Read the model definition and answer for the solid it produces. Units are mm, in the model's axes. Face numbers are marked on the shaded views. Coordinates: 2 decimals unless noted, no trailing zeros. Loops run counter-clockwise (first coordinate to the right, second up) from the corner with the lowest first, then second, coordinate; pieces in that order, holes last. Notation, with made-up numbers: M -37,51.25 L -14,51.25 A28 ccw -14,88.25 Z; hole C 46.5,85.5 d10. An arc over 180 degrees is marked long. One line per item, written item: value. Start each with the question number.
1. Determine the mould class of the marked faces 1, 2 and 3 for opening direction X: +X half, -X half, draft (parallel to the pull), parting line (faces both ways), or undercut.
2. The part is cut by section C-C (x = 20). Write down the section's boundary in (y, z).
3. The part is cut by section B-B (x = 65). Write down the section's boundary in (y, z), then the cut area to 3 significant figures.
4. The part is cut by section A-A (y = 1). Write down the section's boundary in (x, z), then the cut area to 3 significant figures.
5. Flat-ended cylindrical pins translate along their axes: pin 1 (1.5 mm diameter, centred on x = 39.5, y = 3.5, fed in from +Z); pin 2 (0.5 mm diameter, centred on y = 1, z = -0.5, fed in from +X); pin 3 (4.5 mm diameter, centred on x = 84.5, z = 7.5, fed in from -Y); pin 4 (5.5 mm diameter, centred on x = 0, z = 0, fed in from +Y). Find the tip coordinate at first contact, or state that the pin passes through.
6. Consider probe 1 along X at (y, z) = (0.75, 4); probe 2 along X at (y, z) = (0.5, 5.5); probe 3 along Y at (x, z) = (1, -3). Determine where each line is inside the solid, lowest interval first.
7. The part is cut by section D-D (z = 9.5). Write down the section's boundary in (x, y), then the cut area to 3 significant figures.
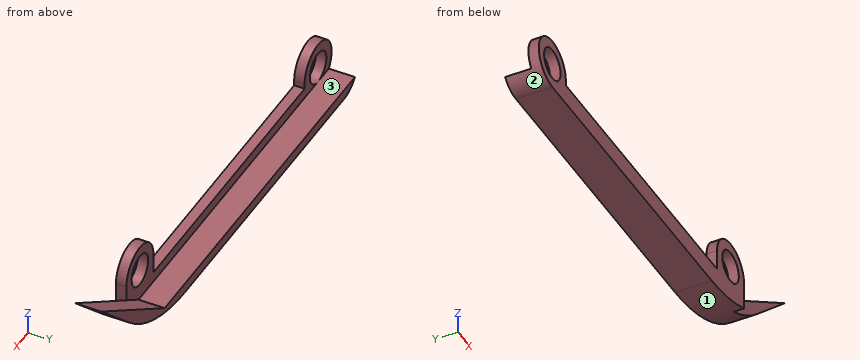
```python
from build123d import *

# Parameters (mm, degrees)
SKETCH1_R           = 3.06
BOSS_EXTRUDE1_DEPTH = 2
BOSS_EXTRUDE2_START = -2
BOSS_EXTRUDE2_DEPTH = 5
SKETCH6_W           = 56
SKETCH6_H           = 2
BOSS_EXTRUDE3_DEPTH = 2
FILLET1_R           = 30
FILLET2_R           = 5


with BuildPart() as part:
    # Sketch1 → Boss-Extrude1 (new body)
    with BuildSketch(Plane(origin=(0, 0, 0), x_dir=(1, 0, 0), z_dir=(0, 1, 0))):
        with BuildLine():
            Line((-5, 0), (-5, 5))
            Line((-5, 5), (71, 5))
            Line((71, 5), (71, -3))
            ThreePointArc((71, -3), (66, -8), (61, -3))
            Line((61, -3), (61, 3.06))
            Line((61, 3.06), (5, 3.06))
            Line((5, 3.06), (5, 0))
            ThreePointArc((5, 0), (0, -5), (-5, 0))
        make_face()
        with Locations(Location((0, 0, 0), (0, 0, 270))):
            Circle(SKETCH1_R, mode=Mode.SUBTRACT)
        with Locations(Location((66, -3, 0), (0, 0, 270))):
            Circle(SKETCH1_R, mode=Mode.SUBTRACT)
    extrude(amount=BOSS_EXTRUDE1_DEPTH)

    # Sketch4 → Boss-Extrude2 (add)
    with BuildSketch(Plane(origin=(0, 0, 0), x_dir=(-1, 0, 0), z_dir=(0, -1, 0)).offset(BOSS_EXTRUDE2_START)):
        Polygon((5, 5), (-71, 5), (-90, -13.010835443), (-66.5, 3.06), (5, 3.06), align=None)
    extrude(amount=-BOSS_EXTRUDE2_DEPTH)

    # Sketch6 → Boss-Extrude3 (add)
    with BuildSketch(Plane(origin=(0, 0, 0), x_dir=(-1, 0, 0), z_dir=(0, -1, 0))):
        with Locations((-33, 2.06)):
            Rectangle(SKETCH6_W, SKETCH6_H)
    extrude(amount=-BOSS_EXTRUDE3_DEPTH)

    # Fillet1
    # the kernel refuses this fillet: 30 mm, written as the material it takes off along each edge
    with BuildSketch(Plane(origin=(71, -27.8984931, -5), x_dir=(0.7257460116750271, 0, 0.6879627363002968), z_dir=(0, 1, 0))) as fillet1_piece_1:
        with BuildLine():
            CenterArc((FILLET1_R * 0.398646574667, -FILLET1_R), FILLET1_R, 90, 43.469057367)
            Line((-FILLET1_R * 0.289316161633, -FILLET1_R * 0.274253988325), (0, 0))
            Line((0, 0), (FILLET1_R * 0.398646574667, 0))
        make_face()
    extrude(amount=64.7969862, mode=Mode.SUBTRACT)

    # Fillet2
    # the kernel refuses this fillet: 5 mm, written as the material it takes off along each edge
    with BuildSketch(Plane(origin=(-5, 19.5, -5), x_dir=(0, 0, 1), z_dir=(0, -1, 0))) as fillet2_piece_1:
        with BuildLine():
            CenterArc((FILLET2_R, -FILLET2_R), FILLET2_R, 90, 90)
            Line((0, -FILLET2_R), (0, 0))
            Line((0, 0), (FILLET2_R, 0))
        make_face()
    extrude(amount=32, mode=Mode.SUBTRACT)


solid = part.part
```
Answer block:
1. face 1: +X half
1. face 2: undercut
1. face 3: draft
2. outline: M 0,-5 L 7,-5 L 7,-3.06 L 2,-3.06 L 2,-1.06 L 0,-1.06 Z
3. outline: M 0,-4.4 L 7,-4.4 L 7,-3.06 L 2,-3.06 L 2,0.11 L 0,0.11 Z; M 0,5.89 L 2,5.89 L 2,7.9 L 0,7.9 Z
3. area: 19.7 mm2
4. outline: M 0,-5 L 59.04,-5 A30 ccw 71,-2.51 L 71,3 A5 ccw 61,3 L 61,-1.06 L 5,-1.06 L 5,0 A5 ccw long Z; hole C 0,0 d6.12; hole C 66,3 d6.12
4. area: 355 mm2
5. pin 1: stops at z = -3.06
5. pin 2: stops at x = 71
5. pin 3: stops at y = 2
5. pin 4: passes through
6. probe 1: x = -3 to 3, 61.1 to 63.11, 68.89 to 70.9
6. probe 2: x = 61.67 to 64.24, 67.76 to 70.33
6. probe 3: y = 0 to 2
7. outline: M 84.87,2 L 86.3,2 L 86.3,7 L 84.87,7 Z
7. area: 7.15 mm2
